from build123d import *

# Parameters (mm, degrees)
SKETCH1_R                        = 15
SKETCH1_R_2                      = 6
SKETCH1_R_3                      = 3.01
BOSS_EXTRUDE4_DEPTH              = 2.54
BOSS_EXTRUDE5_START              = 10
SKETCH1_8_R                      = 6
SKETCH1_8_R_2                    = 3.01
BOSS_EXTRUDE5_DEPTH              = 10
M3_CLEARANCE_HOLE1_D             = 3.4
TAP_DRILL_FOR_M3X0_5_TAP1_REACH  = 30.992
TAP_DRILL_FOR_M3X0_5_TAP1_BORE_R = 1.25
TAP_DRILL_FOR_M3X0_5_TAP2_REACH  = 30.992
TAP_DRILL_FOR_M3X0_5_TAP2_BORE_R = 1.25


with BuildPart() as part:
    # Sketch1 → Boss-Extrude4 (new body)
    # profile 1 of 2: a face of its own
    with BuildSketch(Plane(origin=(0, 0, 0), x_dir=(1, 0, 0), z_dir=(0, 1, 0))):
        with Locations(Location((0, 0, 0), (0, 0, 270))):
            Circle(SKETCH1_R)
        Circle(SKETCH1_R_2, mode=Mode.SUBTRACT)
    # profile 2 of 2: a face of its own
    with BuildSketch(Plane(origin=(0, 0, 0), x_dir=(1, 0, 0), z_dir=(0, 1, 0))):
        Circle(SKETCH1_R_2)
        with Locations(Location((0, 0, 0), (0, 0, 270))):
            Circle(SKETCH1_R_3, mode=Mode.SUBTRACT)
    extrude(amount=-BOSS_EXTRUDE4_DEPTH)

    # Sketch1<8> → Boss-Extrude5 (add)
    with BuildSketch(Plane(origin=(0, 0, 0), x_dir=(1, 0, 0), z_dir=(0, 1, 0)).offset(BOSS_EXTRUDE5_START)):
        with Locations(Location((0, 0, 0), (0, 0, 270))):
            Circle(SKETCH1_8_R)
        with Locations(Location((0, 0, 0), (0, 0, 270))):
            Circle(SKETCH1_8_R_2, mode=Mode.SUBTRACT)
    extrude(amount=-BOSS_EXTRUDE5_DEPTH)

    # M3 Clearance Hole1 (through all)
    with Locations(Plane(origin=(0, 0, 0), x_dir=(1, 0, 0), z_dir=(0, 1, 0))):
        with Locations((0, 12), (12, 0), (-12, 0), (0, -12)):
            Hole(M3_CLEARANCE_HOLE1_D / 2)

    # Tap Drill for M3x0.5 Tap1 bore → Tap Drill for M3x0.5 Tap1 (cut, up to next)
    with BuildSketch(Plane(origin=(-4.242640687, 0, -4.242640687), x_dir=(0, -1, 0), z_dir=(-0.7071067811865464, 0, -0.7071067811865488)), mode=Mode.PRIVATE) as tap_drill_for_m3x0_5_tap1_sk1:
        with Locations((-5, 0)):
            Circle(TAP_DRILL_FOR_M3X0_5_TAP1_BORE_R)
    tap_drill_for_m3x0_5_tap1_tool1 = extrude(tap_drill_for_m3x0_5_tap1_sk1.sketch, amount=-TAP_DRILL_FOR_M3X0_5_TAP1_REACH, mode=Mode.PRIVATE) & part.part
    add(tap_drill_for_m3x0_5_tap1_tool1.solids().sort_by_distance((-4.242641, 5, -4.242641))[0], mode=Mode.SUBTRACT)

    # Tap Drill for M3x0.5 Tap2 bore → Tap Drill for M3x0.5 Tap2 (cut, up to next)
    with BuildSketch(Plane(origin=(-4.242640687, 0, 4.242640687), x_dir=(0, -1, 0), z_dir=(-0.7071067811865512, 0, 0.7071067811865438)), mode=Mode.PRIVATE) as tap_drill_for_m3x0_5_tap2_sk1:
        with Locations((-5, 0)):
            Circle(TAP_DRILL_FOR_M3X0_5_TAP2_BORE_R)
    tap_drill_for_m3x0_5_tap2_tool1 = extrude(tap_drill_for_m3x0_5_tap2_sk1.sketch, amount=-TAP_DRILL_FOR_M3X0_5_TAP2_REACH, mode=Mode.PRIVATE) & part.part
    add(tap_drill_for_m3x0_5_tap2_tool1.solids().sort_by_distance((-4.242641, 5, 4.242641))[0], mode=Mode.SUBTRACT)


solid = part.part
CAD build for the part. Positions are in the model's coordinates, mm. A direction names the side the tool comes from. Give positions to 0.01 mm unless a question says otherwise; leave off trailing zeros. Order: outer loops, then holes, each group sorted by start corner. A loop starts at its lowest first (then second) coordinate and runs counter-clockwise, first axis right, second up. Notation, with made-up numbers: (7.5, -12) -> (61.5, -12) arc R18 ccw to (61.5, 14) -> close; hole circle Ø11 at (25, 4). An arc over 180 degrees is marked (long way). Return JSON: item names as keys, results as strings.
Q1. Saw through at D-D (x = 12). Write the cut outline in (y, z), then the cut area to 3 significant figures.
Working result:
{"outline": "(-2.54, -9) -> (0, -9) -> (0, -1.7) -> (-2.54, -1.7) -> close; (-2.54, 1.7) -> (0, 1.7) -> (0, 9) -> (-2.54, 9) -> close", "area": "37.1 mm²"}
Q2. Saw through at B-B (z = -12). Write the cut outline in (x, y).
Working result:
{"outline": "(-9, -2.54) -> (-1.7, -2.54) -> (-1.7, 0) -> (-9, 0) -> close; (1.7, -2.54) -> (9, -2.54) -> (9, 0) -> (1.7, 0) -> close"}
Q3. Mould opens along Z. For faces 3 (the face through (0.37, -1.29, 13.66)), 4 (the face through (-0.2, 0, 6.5)), 5 (the face through (0.66, -1.252, -14.985)) say: pulls with the +Z half, pulls with the -Z half, needs draft (parallel to the pull), parting line crosses it, or undercut.
Working result:
{"face 3": "undercut", "face 4": "needs draft", "face 5": "parting line crosses it"}
Q4. Saw through at C-C (z = 0). Write the cut outline in (x, y).
Working result:
{"outline": "(-15, -2.54) -> (-13.7, -2.54) -> (-13.7, 0) -> (-15, 0) -> close; (-10.3, -2.54) -> (-3.01, -2.54) -> (-3.01, 10) -> (-6, 10) -> (-6, 0) -> (-10.3, 0) -> close; (3.01, -2.54) -> (10.3, -2.54) -> (10.3, 0) -> (6, 0) -> (6, 10) -> (3.01, 10) -> close; (13.7, -2.54) -> (15, -2.54) -> (15, 0) -> (13.7, 0) -> close"}
Q5. Which spindle directions (+Z, -Z, +X, -X, +Y, -Y) get a long thin tool onto all of the face, cutting with end or side? Do faces 1 (the face through (0.221, -1.288, -13.686)), 2 (the face through (1.802, 5.07, 5.723)). Say none if no direction does.
Working result:
{"face 1": "+Y, -Y", "face 2": "+Y"}
Q6. Flat gauge pin, fed straight in: pin 1 (4 mm diameter, centred on x = -5, z = -9, fed in from +Y). Where does the tip first touch, or does it go through?
Working result:
{"pin 1": "y = 0"}
Q7. Saw through at A-A (x = 0). Write the cut outline in (y, z).
Working result:
{"outline": "(-2.54, -15) -> (0, -15) -> (0, -13.7) -> (-2.54, -13.7) -> close; (-2.54, -10.3) -> (0, -10.3) -> (0, -6) -> (10, -6) -> (10, -3.01) -> (-2.54, -3.01) -> close; (-2.54, 3.01) -> (10, 3.01) -> (10, 6) -> (0, 6) -> (0, 10.3) -> (-2.54, 10.3) -> close; (-2.54, 13.7) -> (0, 13.7) -> (0, 15) -> (-2.54, 15) -> close"}
Q8. Drill centre lines: line 1 (X direction, y = 2.75, z = 0); line 2 (Y direction, x = 6.75, z = -1); line 3 (Z direction, x = 12, y = -1.75). Where is each one in solid material? Low to high.
Working result:
{"line 1": "-6 to -3.01, 3.01 to 6", "line 2": "-2.54 to 0", "line 3": "-9 to -1.7, 1.7 to 9"}
